Autodesk Inventor part; units mm, degrees
ref_plane "YZ Plane" through (0, 0, 0) normal (1, 0, 0) x (0, 1, 0)
ref_plane "XZ Plane" through (0, 0, 0) normal (0, 1, 0) x (-1, 0, 0)
ref_plane "XY Plane" through (0, 0, 0) normal (0, 0, 1) x (1, 0, 0)
sketch "Sketch3" plane through (0, 0, 0) normal (0, 1, 0) x (-1, 0, 0)
  line L0 (105, -125) -> (-105, -125)
  line L1 (-125, -105) -> (-125, 105)
  line L2 (-105, 125) -> (105, 125)
  line L3 (125, 105) -> (125, -105)
  line L4 (125, -125) -> (-125, 125) construction
  line L5 (-125, -125) -> (125, 125) construction
  arc A0 (125, 105) -> (105, 125) centre (105, 105) ccw
  arc A1 (105, -125) -> (125, -105) centre (105, -105) ccw
  arc A2 (-105, 125) -> (-125, 105) centre (-105, 105) ccw
  arc A3 (-125, -105) -> (-105, -125) centre (-105, -105) ccw
  line L6 (-40, 50) -> (40, 50)
  line L7 (50, 40) -> (50, -40)
  line L8 (40, -50) -> (-40, -50)
  line L9 (-50, -40) -> (-50, 40)
  line L10 (-50, 50) -> (50, -50) construction
  line L11 (50, 50) -> (-50, -50) construction
  arc A4 (50, 40) -> (40, 50) centre (40, 40) ccw
  arc A5 (-40, 50) -> (-50, 40) centre (-40, 40) ccw
  arc A6 (-50, -40) -> (-40, -50) centre (-40, -40) ccw
  arc A7 (40, -50) -> (50, -40) centre (40, -40) ccw
  point P0 (0, 0)
  dimension "L0" = 250
  dimension "W0" = 250
  dimension "d126" = 20
  dimension "d127" = 100
  dimension "d128" = 100
  dimension "d129" = 10
extrude "Main Body Extrusion" add sketch "Sketch3" along normal blind 3
sketch "Sketch11" plane through (0, 3, 0) normal (0, 1, 0) x (1, 0, 0)
  circle A0 centre (61.4917, -70.0531) radius 2.5
  circle A1 centre (22.4917, -105.0531) radius 2.5
  circle A2 centre (-22.5083, -70.0531) radius 2.5
  circle A3 centre (-61.5083, -105.0531) radius 2.5
  circle A4 centre (-22.5083, -105.0531) radius 2.5
  circle A5 centre (61.4917, -105.0531) radius 2.5
  circle A6 centre (-61.5083, -70.0531) radius 2.5
  circle A7 centre (61.4917, 104.9469) radius 2.5
  circle A8 centre (61.4917, 69.9469) radius 2.5
  circle A9 centre (22.4917, 104.9469) radius 2.5
  circle A10 centre (-22.5083, 69.9469) radius 2.5
  circle A11 centre (-61.5083, 104.9469) radius 2.5
  circle A12 centre (-22.5083, 104.9469) radius 2.5
  circle A13 centre (22.4917, -70.0531) radius 2.5
  circle A14 centre (22.4917, 69.9469) radius 2.5
  line L0 (-125.0083, 124.9469) -> (124.9917, 124.9469)
  line L1 (124.9917, 124.9469) -> (124.9917, -125.0531)
  line L2 (124.9917, -125.0531) -> (-125.0083, -125.0531)
  line L3 (-125.0083, -125.0531) -> (-125.0083, 124.9469)
  point P0 (0, 0)
  point P1 (-61.5083, 69.9469)
  dimension "d86" = 250
  dimension "d87" = 250
hole "Bracket Holes" at (61.4917, 3, 70.0531) at (22.4917, 3, 105.0531) at (-22.5083, 3, 70.0531) at (-61.5083, 3, 105.0531) at (-22.5083, 3, 105.0531) at (61.4917, 3, 105.0531) at (-61.5083, 3, 70.0531) at (61.4917, 3, -104.9469) at (61.4917, 3, -69.9469) at (22.4917, 3, -104.9469) at (-22.5083, 3, -69.9469) at (-61.5083, 3, -104.9469) at (-22.5083, 3, -104.9469) at (22.4917, 3, 70.0531) at (22.4917, 3, -69.9469) at (-61.5083, 3, -69.9469) direction (0, -1, 0) diameter 5 end through all
sketch "Sketch12" plane through (0, 3, 0) normal (0, 1, 0) x (1, 0, 0)
  line L0 (85, -115) -> (115, -115)
  line L1 (115, -115) -> (115, -110.5263)
  line L2 (105, -105) -> (85, -105)
  line L3 (85, -105) -> (85, -115)
  line L4 (115, -85) -> (105, -85)
  line L5 (105, -85) -> (105, -105)
  line L6 (110.5263, -115) -> (115, -115)
  line L7 (115, -115) -> (115, -85)
  line L8 (125, -105) -> (125, 105)
  line L9 (-105, -125) -> (105, -125)
  line L10 (115, 115) -> (110.5263, 115)
  line L11 (115, 110.5263) -> (115, 115)
  line L12 (105, 105) -> (105, 85)
  line L13 (105, 85) -> (115, 85)
  line L14 (115, 85) -> (115, 115)
  line L15 (85, 115) -> (85, 105)
  line L16 (85, 105) -> (105, 105)
  line L17 (115, 115) -> (85, 115)
  line L18 (-115, 115) -> (-115, 110.5263)
  line L19 (-110.5263, 115) -> (-115, 115)
  line L20 (-105, 105) -> (-85, 105)
  line L21 (-85, 105) -> (-85, 115)
  line L22 (-85, 115) -> (-115, 115)
  line L23 (-115, 85) -> (-105, 85)
  line L24 (-105, 85) -> (-105, 105)
  line L25 (-115, 115) -> (-115, 85)
  line L26 (-115, -115) -> (-110.5263, -115)
  line L27 (-115, -110.5263) -> (-115, -115)
  line L28 (-105, -105) -> (-105, -85)
  line L29 (-105, -85) -> (-115, -85)
  line L30 (-115, -85) -> (-115, -115)
  line L31 (-85, -115) -> (-85, -105)
  line L32 (-85, -105) -> (-105, -105)
  line L33 (-115, -115) -> (-85, -115)
  line L34 (35, -65) -> (65, -65)
  line L35 (65, -65) -> (65, -50.5263)
  line L36 (55, -55) -> (35, -55)
  line L37 (35, -55) -> (35, -65)
  line L38 (65, -35) -> (55, -35)
  line L39 (55, -35) -> (55, -55)
  line L40 (66.4138, -65) -> (65, -65)
  line L41 (65, -65) -> (65, -35)
  line L42 (65, 66.4138) -> (65, 65)
  line L43 (65, 65) -> (50.5263, 65)
  line L44 (65, 65) -> (35, 65)
  line L45 (65, 35) -> (65, 65)
  line L46 (35, 55) -> (55, 55)
  line L47 (55, 55) -> (55, 35)
  line L48 (35, 65) -> (35, 55)
  line L49 (55, 35) -> (65, 35)
  line L50 (-66.4138, 65) -> (-65, 65)
  line L51 (-65, 65) -> (-65, 50.5263)
  line L52 (-65, 65) -> (-65, 35)
  line L53 (-35, 65) -> (-65, 65)
  line L54 (-55, 35) -> (-55, 55)
  line L55 (-55, 55) -> (-35, 55)
  line L56 (-65, 35) -> (-55, 35)
  line L57 (-35, 55) -> (-35, 65)
  line L58 (-65, -66.4138) -> (-65, -65)
  line L59 (-65, -65) -> (-50.5263, -65)
  line L60 (-65, -65) -> (-35, -65)
  line L61 (-65, -35) -> (-65, -65)
  line L62 (-35, -55) -> (-55, -55)
  line L63 (-55, -55) -> (-55, -35)
  line L64 (-35, -65) -> (-35, -55)
  line L65 (-55, -35) -> (-65, -35)
  point P0 (0, 0)
  point P1 (125, -125)
  point P2 (125, 125)
  point P3 (-125, -125)
  point P4 (89, -110)
  point P5 (110, -89)
  point P6 (110, -85)
  point P7 (85, 110)
  point P8 (89, 110)
  point P9 (110, 89)
  point P10 (-110, 85)
  point P11 (-110, 89)
  point P12 (-89, 110)
  point P13 (-85, -110)
  point P14 (-89, -110)
  point P15 (-110, -89)
  point P16 (39, -60)
  point P17 (60, -39)
  point P18 (60, -35)
  point P19 (35, 60)
  point P20 (60, 39)
  point P21 (39, 60)
  point P22 (-60, 35)
  point P23 (-39, 60)
  point P24 (-60, 39)
  point P25 (-35, -60)
  point P26 (-60, -39)
  point P27 (-39, -60)
  dimension "d95" = 30
  dimension "d96" = 30
  dimension "d97" = 20
  dimension "d98" = 20
  dimension "d99" = 10
  dimension "d100" = 10
  dimension "d101" = 4
  dimension "d102" = 5
  dimension "d103" = 5
  dimension "d104" = 4
  dimension "d107" = 360
  dimension "d116" = 30
  dimension "d117" = 30
  dimension "d118" = 20
  dimension "d119" = 20
  dimension "d120" = 4
  dimension "d121" = 5
  dimension "d122" = 5
  dimension "d123" = 4
  dimension "d124" = 60
  dimension "d125" = 60
  dimension "d132" = 360
hole "Hole4" at (89, 3, 110) at (110, 3, 89) at (89, 3, -110) at (110, 3, -89) at (-110, 3, -89) at (-89, 3, -110) at (-89, 3, 110) at (-110, 3, 89) at (-60, 3, 39) at (-39, 3, 60) at (-60, 3, -39) at (-39, 3, -60) at (39, 3, -60) at (60, 3, -39) at (60, 3, 39) at (39, 3, 60) direction (0, -1, 0) diameter 5 end through all
properties part number "L1 Wood Base Iteration 1" material "Aluminum 6061"
Here's how the part is built. I have some questions about the finished solid (model axes, mm). A direction names the side the tool comes from. Coordinates: 2 decimals unless noted, no trailing zeros. Write each loop counter-clockwise with the first axis right and the second up, starting at its lowest first coordinate (ties: lowest second). Pieces come first, ordered by that corner, then holes.
Item 1: I want a section at A-A on x = 0.5. Write out the boundary of the cut face in (y, z).
Item 2: On a 3-axis mill with a long thin cutter (end or side, diameter ignored), from which of +Z, -Z, +X, -X, +Y, -Y can I reach the whole of each face in a straight line? I mean faces 4 (the cylindrical face through (-119.297, 1.479, -118.986)), 5 (the cylindrical face through (-46.99, 1.48, 47.15)). Say none if no direction works.
Item 3: I want a section at C-C on y = 1.2. Count the separate pieces of the cut face and the enclosed holes in it, and give its area (3 significant figures).
Item 4: I want a section at B-B on z = 11. Write out the boundary of the cut face in (x, y), and give its area (3 significant figures).
Item 5: Will this pin go through, and if not, where does the flat tip stop? pin 1 (4.5 mm diameter, centred on x = 39, z = 60, fed in from -Y).
Item 6: If we mould it in two halves opening along Z, with no side actions, what happens to faces 1 (the flat face through (-54, 0, 2)), 2 (the cylindrical face through (-47.15, 1.48, -46.99)), 3 (the cylindrical face through (-118.986, 1.479, 119.297))? For each: +Z half, -Z half, draft (parallel to the pull), parting line (faces both ways), or undercut.
Item 7: If I drill on line 1 (Z direction, x = 89, y = 1.15); line 2 (X direction, y = 2.2, z = -29), over which ranges is the centre line in solid material (lowest first)?
Findings below:
1. outline: (0, -125) - (3, -125) - (3, -50) - (0, -50) - close; (0, 50) - (3, 50) - (3, 125) - (0, 125) - close
2. face 4: -Z, -X, +Y, -Y
2. face 5: +Y, -Y
3. separate pieces: 1
3. enclosed holes: 33
3. area: 51,600 mm2
4. outline: (-125, 0) - (-50, 0) - (-50, 3) - (-125, 3) - close; (50, 0) - (125, 0) - (125, 3) - (50, 3) - close
4. area: 450 mm2
5. pin 1: passes through
6. face 1: draft
6. face 2: undercut
6. face 3: +Z half
7. line 1: z = -125 to -112.5, -107.5 to 107.5, 112.5 to 125
7. line 2: x = -125 to -50, 50 to 125
